Check sheet for the modelled part. Datum: model origin and axes. Units: mm. A direction names the side the tool comes from. Round coordinates to 2 decimals unless told otherwise and drop trailing zeros. Write each loop counter-clockwise with the first axis right and the second up, starting at its lowest first coordinate (ties: lowest second). Pieces come first, ordered by that corner, then holes. Notation, with made-up numbers: (-27.5, -29.5) - (29.5, -29.5) arc R32 ccw to (29.5, 0.5) - close; hole circle Ø9 at (56.5, -15). An arc over 180 degrees is marked (long way). Answer as a JSON object with one key per item and string values. Group by question number.
Item 1: Thickness scan on line 1 (Z direction, x = -10.5, y = 1.3); line 2 (Z direction, x = 9, y = 0.4); line 3 (X direction, y = 1.3, z = 3.75). Record the ranges inside material, lowest first.
Item 2: Set-up check for faces 5 (the cylindrical face through (5.16, 0.74, 7.84)), 6 (the flat face through (38, 0, 0)): record each of +Z, -Z, +X, -X, +Y, -Y from which the full face is reachable in a straight line by a thin tool's end or side.
Item 3: Sectioned sample at B-B on z = -1. Record the boundary of the cut face in (x, y).
Item 4: Release check for a two-part mould opening along Z. For faces 1 (the flat face through (38, 5, 0)), 2 (the flat face through (4, 1.5, -1)), 3 (the flat face through (39.44, 2.465, -12.535)), 4 (the cylindrical face through (90, 2, 0)) record: pulls with the +Z half, pulls with the -Z half, needs draft (parallel to the pull), parting line crosses it, or undercut.
Item 5: Sectioned sample at A-A on x = 5.2. Record the boundary of the cut face in (y, z) (3 decimals).
Item 6: Sectioned sample at C-C on y = 2.6. Record the boundary of the cut face in (x, z), plus the area to 3 significant figures.
Item 7: Gauge pin test, flat ends, axial feed: P1, Ø1, axis at y = 1.5, z = 6, coming from the -X side; P2, Ø3, axis at x = 13.5, z = 9, coming from the -Y side; P3, Ø1.2, axis at y = 1, z = -5.5, coming from the -X side; P4, Ø3, axis at y = 1.5, z = -10.5, coming from the -X side. Record the tip position at first contact, or that the pin passes through.
Item 8: Sectioned sample at D-D on x = 60. Record the boundary of the cut face in (y, z).
```python
from build123d import *

# Parameters (mm, degrees)
BOSS_EXTRUDE1_DEPTH = 5
CUT_EXTRUDE1_DEPTH  = 1.5


with BuildPart() as part:
    # Sketch1 → Boss-Extrude1 (new body)
    with BuildSketch(Plane(origin=(0, 0, 0), x_dir=(1, 0, 0), z_dir=(0, 1, 0))):
        with BuildLine():
            Line((0, 15), (80, 10))
            ThreePointArc((80, 10), (90, 0), (80, -10))
            Line((80, -10), (0, -15))
            ThreePointArc((0, -15), (-15, 0), (0, 15))
        make_face()
    extrude(amount=BOSS_EXTRUDE1_DEPTH)

    # Sketch1<3> → Cut-Extrude1 (cut)
    with BuildSketch(Plane(origin=(0, 0, 0), x_dir=(1, 0, 0), z_dir=(0, 1, 0))):
        with BuildLine():
            Line((3.3, 7.559743015), (3.3, 4.259743015))
            Line((3.3, 4.259743015), (-11.694677741, 2.297056223))
            ThreePointArc((-11.694677741, 2.297056223), (-13, 0.809743015), (-11.694677741, -0.677570192))
            Line((-11.694677741, -0.677570192), (3.3, -2.640256985))
            Line((3.3, -2.640256985), (3.3, -5.940256985))
            ThreePointArc((3.3, -5.940256985), (5.2, -7.840256985), (7.1, -5.940256985))
            Line((7.1, -5.940256985), (7.1, -2.090256985))
            Line((7.1, -2.090256985), (20.062072923, -0.681475402))
            ThreePointArc((20.062072923, -0.681475402), (21.4, 0.809743015), (20.062072923, 2.300961432))
            Line((20.062072923, 2.300961432), (7.1, 3.709743015))
            Line((7.1, 3.709743015), (7.1, 7.559743015))
            ThreePointArc((7.1, 7.559743015), (5.2, 9.459743015), (3.3, 7.559743015))
        make_face()
    extrude(amount=CUT_EXTRUDE1_DEPTH, mode=Mode.SUBTRACT)


solid = part.part
```
Completed:
{
 "1": {"line 1": "-10.71 to -2.45, 0.83 to 10.71", "line 2": "-14.44 to -3.5, 1.88 to 14.44", "line 3": "-14.52 to 3.3, 7.1 to 89.27"},
 "2": {"face 5": "-Y", "face 6": "+Z, -Z, +X, -X, -Y"},
 "3": {"outline": "(-14.97, 0) - (-12.99, 0) - (-12.99, 1.5) - (21.39, 1.5) - (21.39, 0) - (89.95, 0) - (89.95, 5) - (-14.97, 5) - close"},
 "4": {"face 1": "needs draft", "face 2": "undercut", "face 3": "pulls with the -Z half", "face 4": "parting line crosses it"},
 "5": {"outline": "(0, -14.675) - (5, -14.675) - (5, 14.675) - (0, 14.675) - (0, 7.84) - (1.5, 7.84) - (1.5, -9.46) - (0, -9.46) - close"},
 "6": {"outline": "(0, -15) - (80, -10) arc R10 ccw to (80, 10) - (0, 15) arc R15 ccw to start", "area": "2,510 mm²"},
 "7": {"P1": "x = -13.96", "P2": "y = 0", "P3": "x = -14.18", "P4": "x = -12"},
 "8": {"outline": "(0, -11.25) - (5, -11.25) - (5, 11.25) - (0, 11.25) - close"}
}
